Check sheet for the modelled part. Datum: model origin and axes. Units: mm. A direction names the side the tool comes from. Round coordinates to 2 decimals unless told otherwise and drop trailing zeros. Order: outer loops, then holes, each group sorted by start corner. A loop starts at its lowest first (then second) coordinate and runs counter-clockwise, first axis right, second up.
(1) Tool access check on faces 5 (the flat face through (-29.7, -20, 74)), 6 (the flat face through (-27, 3.5, 84)), 7 (the flat face through (-17, -37.1, 46)). Record the directions out of +Z, -Z, +X, -X, +Y, -Y that give a thin tool (end or side, any length) a straight path to the whole face; none if there is none.
(2) Depth check by flat-ended pin: pin 1 (21.5 mm diameter, centred on y = -18.5, z = 18.5, fed in from +X); pin 2 (12 mm diameter, centred on y = -23.5, z = 72.5, fed in from -X); pin 3 (13 mm diameter, centred on x = -27, z = 47, fed in from -Y); pin 4 (4 mm diameter, centred on x = -37.5, y = -35, fed in from -Z). Enter the tip coordinate at first touch or a pass-through.
(3) Sectioned sample at A-A, the plane x = -5.5. Enter the section's corners in (y, z), and give its area (3 significant figures).
(4) Sectioned sample at C-C, the plane z = 57.5. Enter the section's corners in (x, y), and give its area (3 significant figures).
(5) Mould release check, pull along X, two halves, no side actions. Record for faces 1 (the cylindrical face through (-24.689, 1.774, 82.555)), 2 (the cylindrical face through (-29.75, -19.93, 53.76)), 3 (the cylindrical face through (-1.119, -19.444, 10.947)), 4 (the flat face through (-41.76, -20, 16)): released by +X, released by -X, zero draft, split by the parting line, or undercut.
(6) Sectioned sample at D-D, the plane x = -10.5. Enter the section's corners in (y, z).
(7) Thickness scan on probe 1 along Y at (x, z) = (-9.5, 56.5); probe 2 along X at (y, z) = (-1.1, 89.68); probe 3 along X at (y, z) = (-8, 66.5). Record the ranges inside material, lowest first.
```python
from build123d import *

# Parameters (mm, degrees)
ESQUISSE1_W                 = 44.03
ESQUISSE1_H                 = 39.37
BOSS_EXTRU_1_DEPTH          = 93.38
ESQUISSE2_W                 = 12.06
ESQUISSE2_H                 = 39.7
ENL_V_MAT_EXTRU_1_DEPTH     = 93.38
ENL_V_START                 = -68.526093067
ENL_V_MAT_EXTRU_2_OUTLINE_W = 39.37
ENL_V_MAT_EXTRU_2_OUTLINE_H = 28.461412473
ENL_V_MAT_EXTRU_2_DEPTH     = 16.822144735
ESQUISSE4_W                 = 39.49
ESQUISSE4_H                 = 34.83
ENL_V_MAT_EXTRU_3_DEPTH     = 27.4
ESQUISSE5_W                 = 27.43
ESQUISSE5_H                 = 34.83
ENL_V_MAT_EXTRU_4_DEPTH     = 100
ENL_V_START_2               = -2.27
ESQUISSE6_W                 = 28.461412473
ESQUISSE6_H                 = 34.83
ENL_V_MAT_EXTRU_7_DEPTH     = 20
CONG_2_R                    = 10
ESQUISSE7_R                 = 3
BOSS_EXTRU_2_DEPTH          = 3.5
BOSS_EXTRU_3_START          = 3.5
ESQUISSE8_R                 = 3
BOSS_EXTRU_3_DEPTH          = 3.5
ESQUISSE9_R                 = 1.6
ENL_V_MAT_EXTRU_8_DEPTH     = 3.5
ESQUISSE10_RX               = 20.1
ESQUISSE10_RY               = 10.05
ENL_V_MAT_EXTRU_9_DEPTH     = 100
ESQUISSE12_R                = 10.95
ENL_V_MAT_EXTRU_10_DEPTH    = 100


with BuildPart() as part:
    # Esquisse1 → Boss.-Extru.1 (new body)
    with BuildSketch(Plane.XY):
        with Locations((-22.015, -19.685)):
            Rectangle(ESQUISSE1_W, ESQUISSE1_H)
    extrude(amount=BOSS_EXTRU_1_DEPTH)

    # Esquisse2 → Enlèv. mat.-Extru.1 (cut)
    with BuildSketch(Plane(origin=(0, 0, 0), x_dir=(1, 0, 0), z_dir=(0, 1, 0))):
        with Locations((-38, -73.53)):
            Rectangle(ESQUISSE2_W, ESQUISSE2_H)
    extrude(amount=-ENL_V_MAT_EXTRU_1_DEPTH, mode=Mode.SUBTRACT)

    # Enlèv. mat.-Extru.2: read off the stored shape, not the designer's step
    # Enlèv. mat.-Extru.2 outline → Enlèv. mat.-Extru.2 (cut)
    with BuildSketch(Plane(origin=(0, 0, 0), x_dir=(0, 1, 0), z_dir=(0.905787793342715, 0, -0.423731605419439)).offset(ENL_V_START)):
        with Locations((-19.685, 20.845283085)):
            Rectangle(ENL_V_MAT_EXTRU_2_OUTLINE_W, ENL_V_MAT_EXTRU_2_OUTLINE_H)
    extrude(amount=ENL_V_MAT_EXTRU_2_DEPTH, mode=Mode.SUBTRACT)

    # Esquisse4 → Enlèv. mat.-Extru.3 (cut)
    with BuildSketch(Plane(origin=(0, 0, 0), x_dir=(-1, 0, 0), z_dir=(0, 0, -1))):
        with Locations((22.015, -19.685)):
            Rectangle(ESQUISSE4_W, ESQUISSE4_H)
    extrude(amount=-ENL_V_MAT_EXTRU_3_DEPTH, mode=Mode.SUBTRACT)

    # Esquisse5 → Enlèv. mat.-Extru.4 (cut)
    with BuildSketch(Plane.XY.offset(93.38)):
        with Locations((-15.985, -19.685)):
            Rectangle(ESQUISSE5_W, ESQUISSE5_H)
    extrude(amount=-ENL_V_MAT_EXTRU_4_DEPTH, mode=Mode.SUBTRACT)

    # Esquisse6 → Enlèv. mat.-Extru.7 (cut)
    with BuildSketch(Plane(origin=(-46.832805267, 0, 21.908597033), x_dir=(0.42373160541943916, 0, 0.9057877933427149), z_dir=(-0.9057877933427149, 0, 0.42373160541943916)).offset(ENL_V_START_2)):
        with Locations((20.845283085, -19.685)):
            Rectangle(ESQUISSE6_W, ESQUISSE6_H)
    extrude(amount=-ENL_V_MAT_EXTRU_7_DEPTH, mode=Mode.SUBTRACT)

    # Congé2
    # the kernel refuses this fillet: 10 mm, written as the material it takes off along each edge
    with BuildSketch(Plane(origin=(-29.7, -37.1, 52.618083786), x_dir=(0, 0, 1), z_dir=(0, 1, 0))) as cong_2_piece_1:
        with BuildLine():
            CenterArc((2.157105836, -10), CONG_2_R, 90, 11.870832878)
            Line((0.10004547, -0.213861709), (0, 0))
            Line((0, 0), (2.157105836, 0))
        make_face()
    extrude(amount=34.83, mode=Mode.SUBTRACT)

    # Esquisse7 → Boss.-Extru.2 (add)
    with BuildSketch(Plane(origin=(0, -39.37, 0), x_dir=(-1, 0, 0), z_dir=(0, -1, 0))):
        with Locations((27.07, -84.38)):
            Circle(ESQUISSE7_R)
    extrude(amount=BOSS_EXTRU_2_DEPTH)

    # Esquisse8 → Boss.-Extru.3 (add)
    with BuildSketch(Plane(origin=(0, 0, 0), x_dir=(1, 0, 0), z_dir=(0, 1, 0)).offset(BOSS_EXTRU_3_START)):
        with Locations(Location((-27.07, -84.38, 0), (0, 0, 180))):
            Circle(ESQUISSE8_R)
    extrude(amount=-BOSS_EXTRU_3_DEPTH)

    # Esquisse9 → Enlèv. mat.-Extru.8 (cut)
    with BuildSketch(Plane(origin=(0, 0, 0), x_dir=(1, 0, 0), z_dir=(0, 1, 0))):
        with Locations(Location((-5.5, -89.68, 0), (0, 0, 180))):
            Circle(ESQUISSE9_R)
    extrude(amount=-ENL_V_MAT_EXTRU_8_DEPTH, mode=Mode.SUBTRACT)

    # Esquisse10 → Enlèv. mat.-Extru.9 (cut)
    with BuildSketch(Plane(origin=(0, 0, 0), x_dir=(1, 0, 0), z_dir=(0, 1, 0))):
        with Locations(Location((-22.015, 0), (0, 0, -90))):
            Ellipse(ESQUISSE10_RX, ESQUISSE10_RY)
    extrude(amount=-ENL_V_MAT_EXTRU_9_DEPTH, mode=Mode.SUBTRACT)

    # Esquisse12 → Enlèv. mat.-Extru.10 (cut)
    with BuildSketch(Plane(origin=(0, 0, 0), x_dir=(0, 0, -1), z_dir=(1, 0, 0))):
        with Locations((0, -19.685)):
            Circle(ESQUISSE12_R)
    extrude(amount=-ENL_V_MAT_EXTRU_10_DEPTH, mode=Mode.SUBTRACT)


solid = part.part
```
Derived:
1. face 5: +Z, -Z
1. face 6: +Z, -Z, +X, -X, +Y
1. face 7: -Z
2. pin 1: stops at x = 0
2. pin 2: stops at x = -31.97
2. pin 3: stops at y = -39.37
2. pin 4: stops at z = 32.23
3. outline: (-39.37, 0) - (-37.1, 0) - (-37.1, 93.38) - (-39.37, 93.38) - close; (-2.27, 0) - (0, 0) - (0, 88.08) - (-2.27, 88.08) - close; (-2.27, 91.28) - (0, 91.28) - (0, 93.38) - (-2.27, 93.38) - close
3. area: 417 mm2
4. outline: (-31.97, -39.37) - (0, -39.37) - (0, 0) - (-31.97, 0) - close; hole (-29.7, -37.1) - (-2.27, -37.1) - (-2.27, -2.27) - (-29.7, -2.27) - close
4. area: 303 mm2
5. face 1: split by the parting line
5. face 2: undercut
5. face 3: zero draft
5. face 4: undercut
6. outline: (-39.37, 0) - (-37.1, 0) - (-37.1, 93.38) - (-39.37, 93.38) - close; (-2.27, 0) - (0, 0) - (0, 93.38) - (-2.27, 93.38) - close
7. probe 1: y = -39.37 to -37.1, -2.27 to 0
7. probe 2: x = -31.97 to -7.1, -3.9 to 0
7. probe 3: x = -31.97 to -29.7, -2.27 to 0
